CAD build for the part. Positions are in the model's coordinates, mm. Face numbers are marked on the shaded views. A direction names the side the tool comes from. Give positions to 0.01 mm unless a question says otherwise; leave off trailing zeros. Write each loop counter-clockwise with the first axis right and the second up, starting at its lowest first coordinate (ties: lowest second). Pieces come first, ordered by that corner, then holes. Notation, with made-up numbers: (83.5, -4) -> (93.5, -4) arc R12 ccw to (93.5, 8) -> close; hole circle Ø11 at (75.25, 65). An arc over 180 degrees is marked (long way). Answer as a JSON object with one key per item and string values.
```python
from build123d import *

# Parameters (mm, degrees)
F1_DEPTH       = 6
F2_D           = 3.1
F2_CBORE_D     = 5.9
F2_CBORE_DEPTH = 3
F3_D           = 3.1
F3_CBORE_D     = 5.9
F3_CBORE_DEPTH = 3
F5_D           = 3
F5_DEPTH       = 12
F5_TIP         = 0.9012909285


with BuildPart() as f1:
    # F0 (on Front) → F1 (new body)
    with BuildSketch(Plane.XZ):
        with BuildLine():
            ThreePointArc((6.35, 37), (1.8598719395, 35.1401280605), (0, 30.65))
            Line((0, 30.65), (0, 0))
            Line((0, 0), (11.5219274306, 0))
            ThreePointArc((11.5219274306, 0), (15.4558473407, -1.8583173487), (18.1600000875, 1.55))
            Line((18.1600000875, 1.55), (18.1600000875, 8.5))
            Line((18.1600000875, 8.5), (15, 8.5))
            ThreePointArc((15, 8.5), (13.9393398282, 8.9393398282), (13.5, 10))
            Line((13.5, 10), (13.5, 30.65))
            ThreePointArc((13.5, 30.65), (11.6401280605, 35.1401280605), (7.15, 37))
            Line((7.15, 37), (6.35, 37))
        make_face()
    extrude(amount=-F1_DEPTH)

    # F2 (through all)
    with Locations(Plane.XZ):
        with Locations((6.7500000875, 32.11)):
            CounterBoreHole(F2_D / 2, F2_CBORE_D / 2, F2_CBORE_DEPTH)

    # F3 (through all)
    with Locations(Plane.XZ):
        with Locations((14.6600000875, 1.55)):
            CounterBoreHole(F3_D / 2, F3_CBORE_D / 2, F3_CBORE_DEPTH)

    # F5
    with Locations(Plane(origin=(0, 0, 0), x_dir=(0, -1, 0), z_dir=(-1, 0, 0))):
        with Locations((-3, 18)):
            Hole(F5_D / 2, depth=F5_DEPTH)
            with Locations((0, 0, -(F5_DEPTH + F5_TIP / 2))):  # 118° drill point
                Cone(0, F5_D / 2, F5_TIP, mode=Mode.SUBTRACT)


solid = f1.part
```
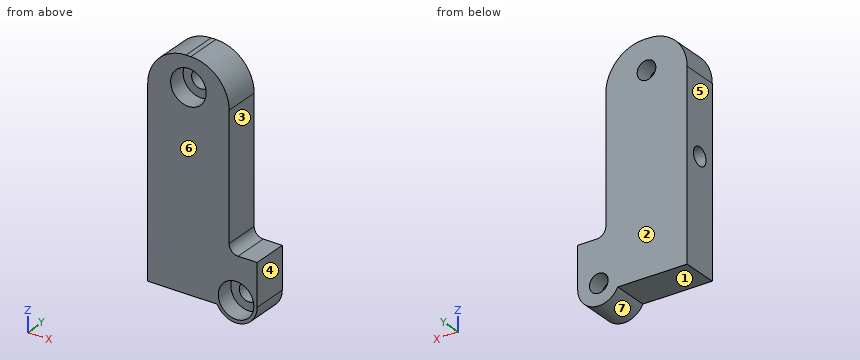
1) Slice it at C-C (y = 0.5). List the corners of the cut face in (x, z).
Model answer:
{"outline": "(0, 0) -> (11.52, 0) arc R3.5 ccw to (18.16, 1.55) -> (18.16, 8.5) -> (15, 8.5) arc R1.5 cw to (13.5, 10) -> (13.5, 30.65) arc R6.35 ccw to (7.15, 37) -> (6.35, 37) arc R6.35 ccw to (0, 30.65) -> close; hole circle Ø5.9 at (6.75, 32.11); hole circle Ø5.9 at (14.66, 1.55)"}
2) 3-axis set-ups, long thin cutter, end or side, ignore diameter. For the marked faces 1, 2 and 3: which of +Z, -Z, +X, -X, +Y, -Y reach the whole face in a straight line?
Model answer:
{"face 1": "-Z, -X, +Y, -Y", "face 2": "+Z, -Z, +X, -X, +Y", "face 3": "+Z, +X, +Y, -Y"}
3) Slice it at A-A (x = 6.75). List the corners of the cut face in (y, z), then the cut area to 3 significant figures.
Model answer:
{"outline": "(0, 0) -> (6, 0) -> (6, 30.56) -> (3, 30.56) -> (3, 29.16) -> (0, 29.16) -> close; (0, 35.06) -> (3, 35.06) -> (3, 33.66) -> (6, 33.66) -> (6, 37) -> (0, 37) -> close; hole circle Ø3 at (3, 18)", "area": "188 mm2"}
4) Mould opens along X. For the marked faces 4, 5, 6 and 7 say: released by +X, released by -X, zero draft, split by the parting line, or undercut.
Model answer:
{"face 4": "released by +X", "face 5": "released by -X", "face 6": "zero draft", "face 7": "split by the parting line"}
5) Slice it at D-D (x = 17). List the corners of the cut face in (y, z), then the cut area to 3 significant figures.
Model answer:
{"outline": "(0, -1.05) -> (6, -1.05) -> (6, 8.5) -> (0, 8.5) -> (0, 3.35) -> (3, 3.35) -> (3, -0.25) -> (0, -0.25) -> close", "area": "46.5 mm2"}
6) Pin check, flat tips, straight feed: pin 1 (2 mm diameter, centred on x = 13.5, y = 2.5, fed in from -Z); pin 2 (2 mm diameter, centred on x = 14, y = 1.5, fed in from +Z); pin 3 (2.5 mm diameter, centred on x = 17, y = 4, fed in from +Z). Stop position of each tip, or through.
Model answer:
{"pin 1": "stops at z = -1.95", "pin 2": "stops at z = 33.12", "pin 3": "stops at z = 8.5"}
7) Slice it at B-B (y = 4.95). List the corners of the cut face in (x, z), then the cut area to 3 significant figures.
Model answer:
{"outline": "(0, 0) -> (11.52, 0) arc R3.5 ccw to (18.16, 1.55) -> (18.16, 8.5) -> (15, 8.5) arc R1.5 cw to (13.5, 10) -> (13.5, 30.65) arc R6.35 ccw to (7.15, 37) -> (6.35, 37) arc R6.35 ccw to (0, 30.65) -> close; hole circle Ø3.1 at (6.75, 32.11); hole circle Ø3.1 at (14.66, 1.55)", "area": "516 mm2"}
8) Wall check: probe 1 along Y at (x, z) = (5.25, 18); probe 2 along Z at (x, y) = (6, 4.05); probe 3 along X at (y, z) = (5.65, 16). Give the ranges that are in metal, low to high.
Model answer:
{"probe 1": "y = 0 to 1.5, 4.5 to 6", "probe 2": "z = 0 to 16.93, 19.07 to 30.75, 33.47 to 36.99", "probe 3": "x = 0 to 13.5"}
